Design review of the part built by this model. Coordinates are the model's own, in mm. Face numbers are marked on the shaded views. A direction names the side the tool comes from. Round coordinates to 2 decimals unless told otherwise and drop trailing zeros. Loops run counter-clockwise (first coordinate to the right, second up) from the corner with the lowest first, then second, coordinate; pieces in that order, holes last. Notation, with made-up numbers: (-7, 52.25) -> (50, 52.25) arc R17 cw to (50, 76.25) -> close; hole circle Ø4 at (27, -14). An arc over 180 degrees is marked (long way). Use a Markdown table: item, result. Add a question column.
from build123d import *

# Parameters (mm, degrees)
SKETCH2_R           = 5
SKETCH2_R_2         = 1.5
SKETCH2_R_3         = 4
BOSS_EXTRUDE1_DEPTH = 6
SKETCH3_R           = 3.5
CUT_EXTRUDE3_DEPTH  = 3
SKETCH4_R           = 4
CUT_EXTRUDE4_DEPTH  = 4


with BuildPart() as part:
    # Sketch2 → Boss-Extrude1 (new body)
    with BuildSketch(Plane(origin=(0, 0, 0), x_dir=(1, 0, 0), z_dir=(0, 1, 0))):
        with Locations((-13.856406461, 10.5)):
            Circle(SKETCH2_R)
        with Locations((-13.856406461, 10.5)):
            Circle(SKETCH2_R_2, mode=Mode.SUBTRACT)
        with Locations((13.856406461, 10.5)):
            Circle(SKETCH2_R)
        with Locations((13.856406461, 10.5)):
            Circle(SKETCH2_R_2, mode=Mode.SUBTRACT)
        with Locations((13.856406461, -10.5)):
            Circle(SKETCH2_R)
        with Locations((13.856406461, -10.5)):
            Circle(SKETCH2_R_2, mode=Mode.SUBTRACT)
        with Locations((-13.856406461, -10.5)):
            Circle(SKETCH2_R)
        with Locations((-13.856406461, -10.5)):
            Circle(SKETCH2_R_2, mode=Mode.SUBTRACT)
        Polygon((17.320508076, 0), (8.660254038, 15), (-8.660254038, 15), (-17.320508076, 0), (-8.660254038, -15), (8.660254038, -15), align=None)
        Circle(SKETCH2_R_3, mode=Mode.SUBTRACT)
        with Locations((8.5, 0)):
            Circle(SKETCH2_R_2, mode=Mode.SUBTRACT)
        with Locations((-8.5, 0)):
            Circle(SKETCH2_R_2, mode=Mode.SUBTRACT)
    extrude(amount=BOSS_EXTRUDE1_DEPTH)

    # Sketch3 → Cut-Extrude3 (cut)
    with BuildSketch(Plane.XZ):
        with Locations((-8.5, 0)):
            Circle(SKETCH3_R)
        with Locations((8.5, 0)):
            Circle(SKETCH3_R)
    extrude(amount=-CUT_EXTRUDE3_DEPTH, mode=Mode.SUBTRACT)

    # Sketch4 → Cut-Extrude4 (cut)
    with BuildSketch(Plane(origin=(0, 6, 0), x_dir=(1, 0, 0), z_dir=(0, 1, 0))):
        with Locations((-13.856406461, 10.5)):
            Circle(SKETCH4_R)
        with Locations((13.856406461, 10.5)):
            Circle(SKETCH4_R)
        with Locations((-13.856406461, -10.5)):
            Circle(SKETCH4_R)
        with Locations((13.856406461, -10.5)):
            Circle(SKETCH4_R)
    extrude(amount=-CUT_EXTRUDE4_DEPTH, mode=Mode.SUBTRACT)


solid = part.part
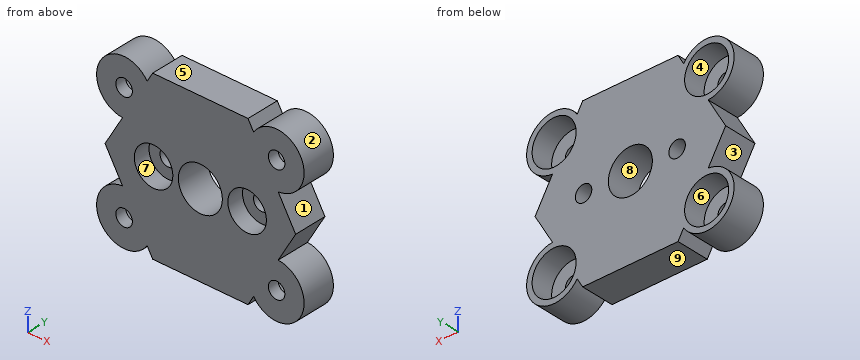
1. For the marked faces 5, 6, 7, 8 and 9, list the 3-axis set-ups (+Z, -Z, +X, -X, +Y, -Y) from which the entire face can be reached by the end or side of a thin tool; tool diameter is ignored.
2. Consider section A-A on z = 10.5. State the section outline as (x, y) points.
3. Consider section B-B on y = 3.5. State the section outline as (x, z) points.
4. Mouldability with a two-part tool opening along X and no side actions: class the marked faces 1, 2, 3 and 4 as +X half, -X half, draft (parallel to the pull), parting line (faces both ways), or undercut.
5. Consider section D-D on x = 11.5. State the section outline as (y, z) points, plus the area to 3 significant figures.
6. Insertion check: P1, Ø4, axis at x = 13.86, z = -10.5, coming from the +Y side; P2, Ø1.8, axis at x = -8.5, z = 0, coming from the +Y side; P3, Ø1, axis at y = 1.5, z = 9.5, coming from the +X side. Each pin has a flat end and moves straight along its axis. Give the tip position at first contact, or say it passes through.
7. Consider section C-C on z = 1. State the section outline as (x, y) points, plus the area to 3 significant figures.
8. To check wall thickness, follow probe 1 along X at (y, z) = (4.5, 0); probe 2 along X at (y, z) = (1.3, 10.5); probe 3 along Z at (x, y) = (-16, 1.9). State the ranges of each line that lie inside material, in increasing order. Write a range as from..to.
Verdict:
| question | item | result |
|---|---|---|
| 1 | face 5 | +Z, +Y, -Y |
| 1 | face 6 | +Y |
| 1 | face 7 | -Y |
| 1 | face 8 | +Y, -Y |
| 1 | face 9 | -Z, +Y, -Y |
| 2 | outline | (-18.86, 0) -> (-15.36, 0) -> (-15.36, 2) -> (-17.86, 2) -> (-17.86, 6) -> (-18.86, 6) -> close; (-12.36, 0) -> (12.36, 0) -> (12.36, 2) -> (9.86, 2) -> (9.86, 6) -> (-9.86, 6) -> (-9.86, 2) -> (-12.36, 2) -> close; (15.36, 0) -> (18.86, 0) -> (18.86, 6) -> (17.86, 6) -> (17.86, 2) -> (15.36, 2) -> close |
| 3 | outline | (-17.32, 0) -> (-14.14, -5.51) arc R5 ccw (long way) to (-9.68, -13.24) -> (-8.66, -15) -> (8.66, -15) -> (9.68, -13.24) arc R5 ccw (long way) to (14.14, -5.51) -> (17.32, 0) -> (14.14, 5.51) arc R5 ccw (long way) to (9.68, 13.24) -> (8.66, 15) -> (-8.66, 15) -> (-9.68, 13.24) arc R5 ccw (long way) to (-14.14, 5.51) -> close; hole circle Ø8 at (-13.86, -10.5); hole circle Ø8 at (-13.86, 10.5); hole circle Ø3 at (-8.5, 0); hole circle Ø8 at (0, 0); hole circle Ø3 at (8.5, 0); hole circle Ø8 at (13.86, -10.5); hole circle Ø8 at (13.86, 10.5) |
| 4 | face 1 | +X half |
| 4 | face 2 | undercut |
| 4 | face 3 | -X half |
| 4 | face 4 | undercut |
| 5 | outline | (0, -14.91) -> (6, -14.91) -> (6, -13.73) -> (2, -13.73) -> (2, -7.27) -> (6, -7.27) -> (6, 7.27) -> (2, 7.27) -> (2, 13.73) -> (6, 13.73) -> (6, 14.91) -> (0, 14.91) -> (0, 1.8) -> (3, 1.8) -> (3, -1.8) -> (0, -1.8) -> close |
| 5 | area | 116 mm² |
| 6 | P1 | stops at y = 2 |
| 6 | P2 | passes through |
| 6 | P3 | stops at x = 18.83 |
| 7 | outline | (-16.74, 0) -> (-11.85, 0) -> (-11.85, 3) -> (-9.62, 3) -> (-9.62, 6) -> (-16.74, 6) -> close; (-7.38, 3) -> (-5.15, 3) -> (-5.15, 0) -> (-3.87, 0) -> (-3.87, 6) -> (-7.38, 6) -> close; (3.87, 0) -> (5.15, 0) -> (5.15, 3) -> (7.38, 3) -> (7.38, 6) -> (3.87, 6) -> close; (9.62, 3) -> (11.85, 3) -> (11.85, 0) -> (16.74, 0) -> (16.74, 6) -> (9.62, 6) -> close |
| 7 | area | 101 mm² |
| 8 | probe 1 | x = -17.32..-10, -7..-4, 4..7, 10..17.32 |
| 8 | probe 2 | x = -18.86..-15.36, -12.36..12.36, 15.36..18.86 |
| 8 | probe 3 | z = -15.02..-5.98, -2.29..2.29, 5.98..15.02 |
